CAD build for the part. Positions are in the model's coordinates, mm. A direction names the side the tool comes from. Give positions to 0.01 mm unless a question says otherwise; leave off trailing zeros. Order: outer loops, then holes, each group sorted by start corner. A loop starts at its lowest first (then second) coordinate and runs counter-clockwise, first axis right, second up. Notation, with made-up numbers: (23, 79.25) -> (47, 79.25) arc R27 cw to (47, 101.25) -> close; hole circle Ø6 at (67, 20.5). An arc over 180 degrees is marked (long way). Use one line per item in the form item = value. Start each with the question number.
1) Cut at A-A, the plane y = 15.25. Give the cut face in (x, z), and give its area (3 significant figures).
2) Probe line 1 (X direction, y = 3.5, z = 0); line 2 (X direction, y = 13, z = -1.75); line 3 (Y direction, x = 5.5, z = -4). List the from-to ranges inside material, lowest first.
3) Cut at B-B, the plane y = 5. Give the cut face in (x, z), and give its area (3 significant figures).
4) Mould opens along X. For faces 6 (the face through (-1.172, 2.785, -8.923)), 7 (the face through (-0.95, 13.45, 4.29)), 8 (the face through (-4, 12, -6)) say: pulls with the +X half, pulls with the -X half, needs draft (parallel to the pull), parting line crosses it, or undercut.
5) Tool access for faces 1 (the face through (4, 0, -7)), 2 (the face through (0.33, 4.93, -7.493)), 3 (the face through (2.52, 16.88, 3.4)), 4 (the face through (-1.172, 9.285, -8.923)), 5 (the face through (-8, 6.5, 3)): list every direction of +Z, -Z, +X, -X, +Y, -Y with a clear straight run to the whole face (end or side of a thin tool).
6) Drop flat-ended pins along their axis: P1, Ø5, axis at x = 1, z = 1.5, coming from the +Y side; P2, Ø1, axis at y = 5.5, z = -4, coming from the -X side; P3, Ø0.6, axis at x = -1.5, y = 15.5, coming from the +Z side; P4, Ø0.6, axis at x = -2, y = 15.5, coming from the -Z side. Give the stop position or say it passes through.
from build123d import *

# Parameters (mm, degrees)
FASE1_SIZE                      = 0.25
SCHNITT_LINEAR_AUSTRAGEN1_DEPTH = 18
FASE2_SIZE                      = 0.25
SKIZZE3_R                       = 7.5
SCHNITT_LINEAR_AUSTRAGEN2_DEPTH = 10
SKIZZE5_R                       = 4
SKIZZE4_R                       = 5.890066201


with BuildPart() as part:
    # Skizze1 → Rotation1 (revolve)
    with BuildSketch(Plane.XY):
        Polygon((0, 0), (9, 0), (9, 5.5), (8, 5.5), (8, 6.5), (9, 6.5), (9, 12), (7, 12), (7, 17), (0, 17), (0, 12), (0, 6.5), (0, 5.5), align=None)
    revolve(axis=Axis((0, -292.433279101, 0), (0, 1, 0)))

    # Fase1
    fase1_edges = [part.edges().sort_by_distance(p)[0] for p in [
        (-9, 6.5, 0),
        (-9, 12, 0),
        (-9, 0, 0),
        (-9, 5.5, 0),
    ]]
    chamfer(fase1_edges, length=FASE1_SIZE)

    # Skizze2 → Schnitt-Linear austragen1 (cut, through all)
    with BuildSketch(Plane(origin=(0, 17, 0), x_dir=(1, 0, 0), z_dir=(0, 1, 0))):
        Polygon((2.165063509, -3.75), (4.330127019, 0), (2.165063509, 3.75), (-2.165063509, 3.75), (-4.330127019, 0), (-2.165063509, -3.75), align=None)
    extrude(amount=-SCHNITT_LINEAR_AUSTRAGEN1_DEPTH, mode=Mode.SUBTRACT)

    # Fase2
    fase2_edges = [part.edges().sort_by_distance(p)[0] for p in [
        (0, 17, 3.75),
        (3.247595264, 17, 1.875),
        (3.247595264, 17, -1.875),
        (0, 17, -3.75),
        (-3.247595264, 17, -1.875),
        (-3.247595264, 17, 1.875),
    ]]
    chamfer(fase2_edges, length=FASE2_SIZE)

    # Skizze3 → Schnitt-Linear austragen2 (cut)
    with BuildSketch(Plane(origin=(0, 0, 0), x_dir=(1, 0, 0), z_dir=(0, 1, 0))):
        with Locations(Location((0, 0, 0), (0, 0, 270))):  # turned: the seam where the file's is
            Circle(SKIZZE3_R)
    extrude(amount=SCHNITT_LINEAR_AUSTRAGEN2_DEPTH, mode=Mode.SUBTRACT)

    # Skizze5 → Schnitt-Ausformung2 section 0
    with BuildSketch(Plane(origin=(0, 17, 0), x_dir=(1, 0, 0), z_dir=(0, 1, 0))):
        Circle(SKIZZE5_R)
    # Skizze4 → Schnitt-Ausformung2 section 1
    with BuildSketch(Plane(origin=(0, 0, 0), x_dir=(1, 0, 0), z_dir=(0, 1, 0))):
        Circle(SKIZZE4_R)
    loft(mode=Mode.SUBTRACT)


solid = part.part
Result:
q1.outline = circle Ø14 at (0, 0); hole (-4.33, 0) -> (-4.19, -0.25) arc R4.19 ccw to (-2.31, -3.5) -> (-2.17, -3.75) -> (-1.88, -3.75) arc R4.19 ccw to (1.88, -3.75) -> (2.17, -3.75) -> (2.31, -3.5) arc R4.19 ccw to (4.19, -0.25) -> (4.33, 0) -> (4.19, 0.25) arc R4.19 ccw to (2.31, 3.5) -> (2.17, 3.75) -> (1.88, 3.75) arc R4.19 ccw to (-1.88, 3.75) -> (-2.17, 3.75) -> (-2.31, 3.5) arc R4.19 ccw to (-4.19, 0.25) -> close
q1.area = 98.5 mm²
q2.line_1 = -9 to -7.5, 7.5 to 9
q2.line_2 = -6.78 to -4.09, 4.09 to 6.78
q2.line_3 = 10 to 17
q3.outline = circle Ø18 at (0, 0); hole circle Ø15 at (0, 0)
q3.area = 77.8 mm²
q4.face_6 = parting line crosses it
q4.face_7 = undercut
q4.face_8 = needs draft
q5.face_1 = +Z, -Z, +X, -X, -Y
q5.face_2 = -Y
q5.face_3 = +Y
q5.face_4 = +Y, -Y
q5.face_5 = none
q6.P1 = 17
q6.P2 = -8.26
q6.P3 = 6.9
q6.P4 = -6.79
